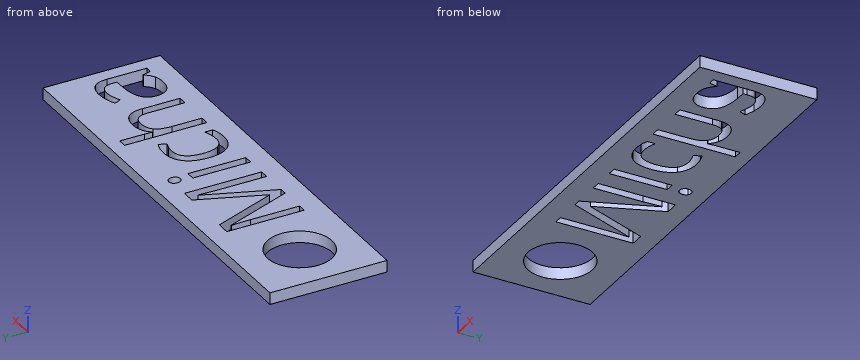
```python
from build123d import *

# Parameters (mm, degrees)
F0_W     = 70
F0_H     = 20
F0_W_2   = 1.5003956149
F0_H_2   = 9.901454684
F2_DEPTH = 2
F3_D     = 11
F3_DEPTH = 17
F3_TIP   = 3.3047334047


with BuildPart() as f2:
    # F0 (on Top) → F2 (new body)
    with BuildSketch(Plane.XY):
        with Locations((-35, 10)):
            Rectangle(F0_W, F0_H)
        with Locations((-33.6410080478, 8.5138517956)):
            Rectangle(F0_W_2, F0_H_2, mode=Mode.SUBTRACT)
        with BuildLine():
            add(Edge.make_bspline(
                [(-23.2524307027, 3.8984729919), (-24.244021639, 3.3809955062), (-25.7530900609, 3.3809955062)],
                knots=[0, 0, 0, 1, 1, 1], degree=2))
            add(Edge.make_bspline(
                [(-25.7530900609, 3.3809955062), (-27.9039462025, 3.3809955062), (-29.0834479575, 4.7050440449)],
                knots=[0, 0, 0, 1, 1, 1], degree=2))
            add(Edge.make_bspline(
                [(-29.0834479575, 4.7050440449), (-30.2629497126, 6.0290925837), (-30.2629497126, 8.4516966786)],
                knots=[0, 0, 0, 1, 1, 1], degree=2))
            add(Edge.make_bspline(
                [(-30.2629497126, 8.4516966786), (-30.2629497126, 10.9350104228), (-29.0646568756, 12.2908592539)],
                knots=[0, 0, 0, 1, 1, 1], degree=2))
            add(Edge.make_bspline(
                [(-29.0646568756, 12.2908592539), (-27.8663640387, 13.6467080851), (-25.654798248, 13.6467080851)],
                knots=[0, 0, 0, 1, 1, 1], degree=2))
            add(Edge.make_bspline(
                [(-25.654798248, 13.6467080851), (-24.9407371365, 13.6467080851), (-24.2266760249, 13.4920430265)],
                knots=[0, 0, 0, 1, 1, 1], degree=2))
            add(Edge.make_bspline(
                [(-24.2266760249, 13.4920430265), (-23.5126149134, 13.337377968), (-23.107883919, 13.1292305994)],
                knots=[0, 0, 0, 1, 1, 1], degree=2))
            Line((-23.107883919, 13.1292305994), (-23.5675426912, 11.8572189028))
            add(Edge.make_bspline(
                [(-23.5675426912, 11.8572189028), (-24.0647836272, 12.0566934643), (-24.651643569, 12.1867855697)],
                knots=[0, 0, 0, 1, 1, 1], degree=2))
            add(Edge.make_bspline(
                [(-24.651643569, 12.1867855697), (-25.2385035109, 12.316877675), (-25.6894894761, 12.316877675)],
                knots=[0, 0, 0, 1, 1, 1], degree=2))
            add(Edge.make_bspline(
                [(-25.6894894761, 12.316877675), (-28.7076263199, 12.316877675), (-28.7076263199, 8.4690422927)],
                knots=[0, 0, 0, 1, 1, 1], degree=2))
            add(Edge.make_bspline(
                [(-28.7076263199, 8.4690422927), (-28.7076263199, 6.6448618823), (-27.9718831908, 5.6691710923)],
                knots=[0, 0, 0, 1, 1, 1], degree=2))
            add(Edge.make_bspline(
                [(-27.9718831908, 5.6691710923), (-27.2361400617, 4.6934803022), (-25.7906722247, 4.6934803022)],
                knots=[0, 0, 0, 1, 1, 1], degree=2))
            add(Edge.make_bspline(
                [(-25.7906722247, 4.6934803022), (-24.5533517561, 4.6934803022), (-23.2524307027, 5.2254124663)],
                knots=[0, 0, 0, 1, 1, 1], degree=2))
            Line((-23.2524307027, 5.2254124663), (-23.2524307027, 3.8984729919))
        make_face(mode=Mode.SUBTRACT)
        with BuildLine():
            Line((-2.3451839072, 3.5631244536), (-3.4581941418, 3.5631244536))
            Line((-3.4581941418, 3.5631244536), (-3.7559605162, 4.9739010626))
            Line((-3.7559605162, 4.9739010626), (-3.8282339081, 4.9739010626))
            add(Edge.make_bspline(
                [(-3.8282339081, 4.9739010626), (-4.5683134407, 4.0430197756), (-5.3040565697, 3.7120076409)],
                knots=[0, 0, 0, 1, 1, 1], degree=2))
            add(Edge.make_bspline(
                [(-5.3040565697, 3.7120076409), (-6.0397996988, 3.3809955062), (-7.1441371263, 3.3809955062)],
                knots=[0, 0, 0, 1, 1, 1], degree=2))
            add(Edge.make_bspline(
                [(-7.1441371263, 3.3809955062), (-8.6156233845, 3.3809955062), (-9.4511037943, 4.1413115885)],
                knots=[0, 0, 0, 1, 1, 1], degree=2))
            add(Edge.make_bspline(
                [(-9.4511037943, 4.1413115885), (-10.2865842041, 4.9016276708), (-10.2865842041, 6.3008405371)],
                knots=[0, 0, 0, 1, 1, 1], degree=2))
            add(Edge.make_bspline(
                [(-10.2865842041, 6.3008405371), (-10.2865842041, 9.2987408312), (-5.4905219207, 9.4432876149)],
                knots=[0, 0, 0, 1, 1, 1], degree=2))
            Line((-5.4905219207, 9.4432876149), (-3.810888294, 9.4982153927))
            Line((-3.810888294, 9.4982153927), (-3.810888294, 10.1139846913))
            add(Edge.make_bspline(
                [(-3.810888294, 10.1139846913), (-3.810888294, 11.279031768), (-4.3110201657, 11.8340914174)],
                knots=[0, 0, 0, 1, 1, 1], degree=2))
            add(Edge.make_bspline(
                [(-4.3110201657, 11.8340914174), (-4.8111520373, 12.3891510669), (-5.9154894648, 12.3891510669)],
                knots=[0, 0, 0, 1, 1, 1], degree=2))
            add(Edge.make_bspline(
                [(-5.9154894648, 12.3891510669), (-7.1528099334, 12.3891510669), (-8.7139151974, 11.6317259202)],
                knots=[0, 0, 0, 1, 1, 1], degree=2))
            Line((-8.7139151974, 11.6317259202), (-9.1764649053, 12.7794273829))
            add(Edge.make_bspline(
                [(-9.1764649053, 12.7794273829), (-8.4450581797, 13.1754855702), (-7.5734410739, 13.4009785528)],
                knots=[0, 0, 0, 1, 1, 1], degree=2))
            add(Edge.make_bspline(
                [(-7.5734410739, 13.4009785528), (-6.7018239682, 13.6264715354), (-5.8229795232, 13.6264715354)],
                knots=[0, 0, 0, 1, 1, 1], degree=2))
            add(Edge.make_bspline(
                [(-5.8229795232, 13.6264715354), (-4.0537268907, 13.6264715354), (-3.1994553989, 12.8415824999)],
                knots=[0, 0, 0, 1, 1, 1], degree=2))
            add(Edge.make_bspline(
                [(-3.1994553989, 12.8415824999), (-2.3451839072, 12.0566934643), (-2.3451839072, 10.3221320598)],
                knots=[0, 0, 0, 1, 1, 1], degree=2))
            Line((-2.3451839072, 10.3221320598), (-2.3451839072, 3.5631244536))
        make_face(mode=Mode.SUBTRACT)
        with BuildLine():
            Line((-43.7867467963, 3.5631244536), (-45.0240672648, 3.5631244536))
            Line((-45.0240672648, 3.5631244536), (-49.5050175598, 15.271413934))
            Line((-49.5050175598, 15.271413934), (-49.5772909516, 15.271413934))
            add(Edge.make_bspline(
                [(-49.5772909516, 15.271413934), (-49.450089782, 13.8808738747), (-49.450089782, 11.9641835228)],
                knots=[0, 0, 0, 1, 1, 1], degree=2))
            Line((-49.450089782, 11.9641835228), (-49.450089782, 3.5631244536))
            Line((-49.450089782, 3.5631244536), (-50.869539198, 3.5631244536))
            Line((-50.869539198, 3.5631244536), (-50.869539198, 16.7718095489))
            Line((-50.869539198, 16.7718095489), (-48.5567906586, 16.7718095489))
            Line((-48.5567906586, 16.7718095489), (-44.3736067381, 5.875872993))
            Line((-44.3736067381, 5.875872993), (-44.3013333463, 5.875872993))
            Line((-44.3013333463, 5.875872993), (-40.0834581977, 16.7718095489))
            Line((-40.0834581977, 16.7718095489), (-37.7880552724, 16.7718095489))
            Line((-37.7880552724, 16.7718095489), (-37.7880552724, 3.5631244536))
            Line((-37.7880552724, 3.5631244536), (-39.3231421154, 3.5631244536))
            Line((-39.3231421154, 3.5631244536), (-39.3231421154, 12.0740390784))
            add(Edge.make_bspline(
                [(-39.3231421154, 12.0740390784), (-39.3231421154, 13.5368525295), (-39.1959409457, 15.2540683199)],
                knots=[0, 0, 0, 1, 1, 1], degree=2))
            Line((-39.1959409457, 15.2540683199), (-39.2682143376, 15.2540683199))
            Line((-39.2682143376, 15.2540683199), (-43.7867467963, 3.5631244536))
        make_face(mode=Mode.SUBTRACT)
        with BuildLine():
            Line((-12.6253511645, 3.5631244536), (-14.1257467794, 3.5631244536))
            Line((-14.1257467794, 3.5631244536), (-14.1257467794, 9.9694379076))
            add(Edge.make_bspline(
                [(-14.1257467794, 9.9694379076), (-14.1257467794, 11.1778490194), (-14.6764700254, 11.7748272361)],
                knots=[0, 0, 0, 1, 1, 1], degree=2))
            add(Edge.make_bspline(
                [(-14.6764700254, 11.7748272361), (-15.2271932713, 12.3718054528), (-16.4038040907, 12.3718054528)],
                knots=[0, 0, 0, 1, 1, 1], degree=2))
            add(Edge.make_bspline(
                [(-16.4038040907, 12.3718054528), (-17.9649093547, 12.3718054528), (-18.6833068697, 11.5218703646)],
                knots=[0, 0, 0, 1, 1, 1], degree=2))
            add(Edge.make_bspline(
                [(-18.6833068697, 11.5218703646), (-19.4017043848, 10.6719352764), (-19.4017043848, 8.7407902461)],
                knots=[0, 0, 0, 1, 1, 1], degree=2))
            Line((-19.4017043848, 8.7407902461), (-19.4017043848, 3.5631244536))
            Line((-19.4017043848, 3.5631244536), (-20.9020999997, 3.5631244536))
            Line((-20.9020999997, 3.5631244536), (-20.9020999997, 17.6217446371))
            Line((-20.9020999997, 17.6217446371), (-19.4017043848, 17.6217446371))
            Line((-19.4017043848, 17.6217446371), (-19.4017043848, 13.3662873247))
            add(Edge.make_bspline(
                [(-19.4017043848, 13.3662873247), (-19.4017043848, 12.5972984354), (-19.4739777766, 12.0913846924)],
                knots=[0, 0, 0, 1, 1, 1], degree=2))
            Line((-19.4739777766, 12.0913846924), (-19.3843587707, 12.0913846924))
            add(Edge.make_bspline(
                [(-19.3843587707, 12.0913846924), (-18.9420456126, 12.8054458039), (-18.1239108168, 13.2159586697)],
                knots=[0, 0, 0, 1, 1, 1], degree=2))
            add(Edge.make_bspline(
                [(-18.1239108168, 13.2159586697), (-17.305776021, 13.6264715354), (-16.259257307, 13.6264715354)],
                knots=[0, 0, 0, 1, 1, 1], degree=2))
            add(Edge.make_bspline(
                [(-16.259257307, 13.6264715354), (-14.4437497036, 13.6264715354), (-13.5345504341, 12.7635272367)],
                knots=[0, 0, 0, 1, 1, 1], degree=2))
            add(Edge.make_bspline(
                [(-13.5345504341, 12.7635272367), (-12.6253511645, 11.9005829379), (-12.6253511645, 10.0214747497)],
                knots=[0, 0, 0, 1, 1, 1], degree=2))
            Line((-12.6253511645, 10.0214747497), (-12.6253511645, 3.5631244536))
        make_face(mode=Mode.SUBTRACT)
        with BuildLine():
            add(Edge.make_bspline(
                [(-34.2654501534, 15.3928332323), (-34.5184070249, 15.6414537003), (-34.5184070249, 16.1473674433)],
                knots=[0, 0, 0, 1, 1, 1], degree=2))
            add(Edge.make_bspline(
                [(-34.5184070249, 16.1473674433), (-34.5184070249, 16.6619539933), (-34.2654501534, 16.9019016542)],
                knots=[0, 0, 0, 1, 1, 1], degree=2))
            add(Edge.make_bspline(
                [(-34.2654501534, 16.9019016542), (-34.012493282, 17.1418493152), (-33.630889773, 17.1418493152)],
                knots=[0, 0, 0, 1, 1, 1], degree=2))
            add(Edge.make_bspline(
                [(-33.630889773, 17.1418493152), (-33.2695228137, 17.1418493152), (-33.0078931352, 16.8975652507)],
                knots=[0, 0, 0, 1, 1, 1], degree=2))
            add(Edge.make_bspline(
                [(-33.0078931352, 16.8975652507), (-32.7462634567, 16.6532811862), (-32.7462634567, 16.1473674433)],
                knots=[0, 0, 0, 1, 1, 1], degree=2))
            add(Edge.make_bspline(
                [(-32.7462634567, 16.1473674433), (-32.7462634567, 15.6414537003), (-33.0078931352, 15.3928332323)],
                knots=[0, 0, 0, 1, 1, 1], degree=2))
            add(Edge.make_bspline(
                [(-33.0078931352, 15.3928332323), (-33.2695228137, 15.1442127643), (-33.630889773, 15.1442127643)],
                knots=[0, 0, 0, 1, 1, 1], degree=2))
            add(Edge.make_bspline(
                [(-33.630889773, 15.1442127643), (-34.012493282, 15.1442127643), (-34.2654501534, 15.3928332323)],
                knots=[0, 0, 0, 1, 1, 1], degree=2))
        make_face(mode=Mode.SUBTRACT)
    extrude(amount=-F2_DEPTH)

    # F3
    with Locations(Plane.XY):
        with Locations((-60.7941076159, 9.8129231483)):
            Hole(F3_D / 2, depth=F3_DEPTH)
            with Locations((0, 0, -(F3_DEPTH + F3_TIP / 2))):  # 118° drill point
                Cone(0, F3_D / 2, F3_TIP, mode=Mode.SUBTRACT)


solid = f2.part
```
Here's how the part is built. I have some questions about the finished solid (model axes, mm). Give positions to 0.01 mm unless a question says otherwise; leave off trailing zeros. Loops run counter-clockwise (first coordinate to the right, second up) from the corner with the lowest first, then second, coordinate; pieces in that order, holes last. Notation, with made-up numbers: (81, 21) -> (88, 21) arc R23 cw to (88, 34) -> close; hole circle Ø5 at (-12.5, 5.25). An arc over 180 degrees is marked (long way). Use one line per item in the form item = value. Start each with the question number.
1) Please list where these lines run through material, in increasing order: line 1 along Y through (x, z) = (-4.5, -1.15); line 2 along Y through (x, z) = (-24.5, -1.65); line 3 along Y through (x, z) = (-56, -0.2).
2) Imagine slicing it at A-A (x = -56). Please give me the cut outline in (y, z).
3) Imagine slicing it at B-B (z = -0.6). Count the separate pieces of the cut face and the enclosed holes in it, then the cut area to 3 significant figures.
Check values:
q1.line_1 = 0 to 4.25, 9.48 to 12.01, 13.49 to 20
q1.line_2 = 0 to 3.49, 4.83 to 12.15, 13.55 to 20
q1.line_3 = 0 to 7.12, 12.51 to 20
q2.outline = (0, -2) -> (7.12, -2) -> (7.12, 0) -> (0, 0) -> close; (12.51, -2) -> (20, -2) -> (20, 0) -> (12.51, 0) -> close
q3.separate_pieces = 1
q3.enclosed_holes = 7
q3.area = 1,090 mm^2
